from build123d import *

# Parameters (mm, degrees)
F1_DEPTH = 5.08
F2_R     = 76.2
F2_R_2   = 19.05
F3_DEPTH = 2.54


with BuildPart() as f1:
    # F0 (on Front) → F1 (new body)
    with BuildSketch(Plane.XZ):
        with BuildLine():
            ThreePointArc((1.905, -31.692798), (23.114349, -21.766703), (31.75, 0))
            ThreePointArc((31.75, 0), (23.114054, 21.767016), (1.904143, 31.69285))
            ThreePointArc((1.904143, 31.69285), (0, 29.845), (-1.904143, 31.69285))
            ThreePointArc((-1.904143, 31.69285), (-31.75, 0.000429), (-1.905, -31.692798))
            Line((-1.905, -31.692798), (-1.905, -7.62))
            Line((-1.905, -7.62), (-3.175, -7.62))
            Line((-3.175, -7.62), (-3.175, 7.62))
            ThreePointArc((-3.175, 7.62), (0, 10.795), (3.175, 7.62))
            Line((3.175, 7.62), (3.175, -7.62))
            Line((3.175, -7.62), (1.905, -7.62))
            Line((1.905, -7.62), (1.905, -31.692798))
        make_face()
    extrude(amount=F1_DEPTH)

    # F2 (on face) → F3 (cut)
    with BuildSketch(Plane.XZ.offset(5.08)):
        Circle(F2_R)
        Circle(F2_R_2, mode=Mode.SUBTRACT)
    extrude(amount=-F3_DEPTH, mode=Mode.SUBTRACT)


solid = f1.part
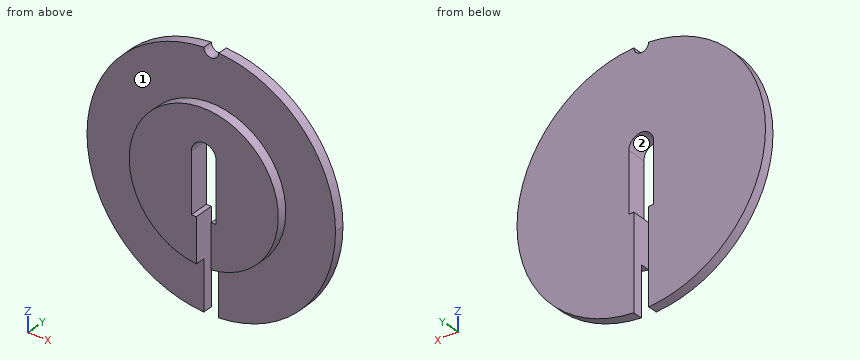
Design review of the part built by this model. Coordinates are the model's own, in mm. Face numbers are marked on the shaded views. Round coordinates to 2 decimals unless told otherwise and drop trailing zeros. Write each loop counter-clockwise with the first axis right and the second up, starting at its lowest first coordinate (ties: lowest second). Pieces come first, ordered by that corner, then holes.
Item 1: Draft analysis for pull direction Z (two halves, no side actions). For the marked faces 1 and 2, state which applies: released by +Z, released by -Z, zero draft, split by the parting line, or undercut.
Item 2: Wall thickness on L1, parallel to Y at x = -23.5, z = -12; L2, parallel to X at y = -1.8, z = -8 (3 decimals); L3, parallel to X at y = -0.85, z = 10: over which ranges is each line inside the solid? List them lowest first.
Item 3: Consider section B-B on x = -11. Give the boundary of the cut face in (y, z), and give its area (3 significant figures).
Item 4: Consider section A-A on z = -9.5. Give the boundary of the cut face in (x, y) (3 decimals).
Item 5: Consider section C-C on y = -0.8. Give the boundary of the cut face in (x, z) (3 decimals), and give its area (3 significant figures).
Item 6: For pin 1 Ø2.5 at (y, z) = (-2.5, -25) entering from -X; pin 2 Ø0.6 at (x, y) = (3, -2) entering from +Z (3 decimals); pin 3 Ø8 at (x, z) = (2, 24) entering from -Y; pin 4 Ø8 at (x, z) = (-12.5, -14.5) entering from +Y, all flat-tipped, find the tip position at first contact; note any pin that passes through.
Item 7: Consider section D-D on z = 18. Give the boundary of the cut face in (x, y).
Check values:
1. face 1: zero draft
1. face 2: undercut
2. L1: y = -2.54 to 0
2. L2: x = -30.726 to -1.905, 1.905 to 30.726
2. L3: x = -30.13 to -2.1, 2.1 to 30.13
3. outline: (-5.08, -15.55) - (-2.54, -15.55) - (-2.54, -29.78) - (0, -29.78) - (0, 29.78) - (-2.54, 29.78) - (-2.54, 15.55) - (-5.08, 15.55) - close
3. area: 230 mm2
4. outline: (-30.295, -2.54) - (-16.512, -2.54) - (-16.512, -5.08) - (-1.905, -5.08) - (-1.905, 0) - (-30.295, 0) - close; (1.905, -5.08) - (16.512, -5.08) - (16.512, -2.54) - (30.295, -2.54) - (30.295, 0) - (1.905, 0) - close
5. outline: (-3.175, -7.62) - (-3.175, 7.62) arc R3.175 cw to (3.175, 7.62) - (3.175, -7.62) - (1.905, -7.62) - (1.905, -31.693) arc R31.75 ccw to (31.75, 0) arc R31.75 ccw to (1.904, 31.693) arc R1.905 cw to (-1.904, 31.693) arc R31.75 ccw to (-1.905, -31.693) - (-1.905, -7.62) - close
5. area: 2,960 mm2
6. pin 1: stops at x = -21.07
6. pin 2: stops at z = 31.635
6. pin 3: stops at y = -2.54
6. pin 4: stops at y = 0
7. outline: (-26.15, -2.54) - (-6.24, -2.54) - (-6.24, -5.08) - (6.24, -5.08) - (6.24, -2.54) - (26.15, -2.54) - (26.15, 0) - (-26.15, 0) - close
